Can you work these out from the model? Positions are in its coordinate system, mm. Face numbers are marked on the shaded views. Coordinates: 2 decimals unless noted, no trailing zeros. Order: outer loops, then holes, each group sorted by start corner. A loop starts at its lowest first (then second) coordinate and runs counter-clockwise, first axis right, second up. Notation, with made-up numbers: M -15,43.5 L -8,43.5 A12 ccw -8,62.5 Z; hole C 77,63 d6. An arc over 180 degrees is marked long. Answer as a JSON object with one key per item and string values.
from build123d import *

# Parameters (mm, degrees)
F0_W          = 3
F0_H          = 9
F0_H_2        = 7
F0_H_3        = 3
F0_R          = 2.1
F0_W_2        = 1
F1_DEPTH      = 2
F2_DEPTH      = 34
F3_W          = 4
F3_H          = 2
F4_DEPTH      = 34
F5_SIZE       = 1.99999
F7_W          = 1
F7_H          = 1
F8_DEPTH      = 1
F3_W_2        = 31
F9_DEPTH      = 10
F10_R         = 1.99999
F11_T1_DEPTH  = 32
F11_T3_DEPTH  = 34.50001
F11_T5_DEPTH  = 32.00001
F11_T7_DEPTH  = 19.5
F11_T9_DEPTH  = 11.5
F11_T11_DEPTH = 44
F11_T13_DEPTH = 36.5
F11_T16_ANGLE = 90
F11_T18_ANGLE = 90
F11_T23_DEPTH = 34.50001
F11_T27_DEPTH = 22
F11_T34_DEPTH = 14
F11_T38_DEPTH = 39
F11_T45_DEPTH = 22
F11_T49_DEPTH = 34.50001


# Not quite as in the source:
# - a fillet or chamfer that OpenCascade refuses, or shapes differently, is made with other operations: its cross-section is extruded or revolved along the edge and cut away or added
# - a fillet or chamfer is up to 0.001 mm smaller than in the source, because OpenCascade refuses the exact size
# - a feature of the source that left no trace in its solid (it failed there, or was rolled back) is left out
# - a feature names something its author has since deleted; it is built from what else it names


with BuildPart() as f1:
    # F0 (on Top) → F1 (new body)
    with BuildSketch(Plane.XY):
        with Locations((18, 20.5)):
            Rectangle(F0_W, F0_H)
        with Locations((-18, 20.5)):
            Rectangle(F0_W, F0_H)
        with Locations((18, -21.5)):
            Rectangle(F0_W, F0_H_2)
        with Locations((-18, -21.5)):
            Rectangle(F0_W, F0_H_2)
        with Locations((18, -16.5)):
            Rectangle(F0_W, F0_H_3)
        with Locations((-18, -16.5)):
            Rectangle(F0_W, F0_H_3)
        Polygon((19.5, -35), (19.5, -25), (16.5, -25), (-16.5, -25), (-19.5, -25), (-19.5, -35), align=None)
        with Locations((0, -30)):
            Circle(F0_R, mode=Mode.SUBTRACT)
        Polygon((19.5, -15), (19.5, 16), (16.5, 16), (16.5, 15), (16.5, -15), align=None)
        Polygon((-16.5, 15), (-16.5, 16), (-19.5, 16), (-19.5, 15), (-19.5, -15), (-16.5, -15), align=None)
        Polygon((16.5, 16), (16.5, 25), (-16.5, 25), (-16.5, 16), (-16.5, 15), (16.5, 15), align=None)
        with Locations((0, 20)):
            Circle(F0_R, mode=Mode.SUBTRACT)
        Polygon((16.5, -15), (16.5, 15), (-16.5, 15), (-16.5, -15), (-15.5, -15), (15.5, -15), align=None)
        with Locations((-16, -16.5)):
            Rectangle(F0_W_2, F0_H_3)
        with Locations((16, -16.5)):
            Rectangle(F0_W_2, F0_H_3)
        Polygon((16.5, -25), (16.5, -18), (15.5, -18), (15.5, -15), (-15.5, -15), (-15.5, -18), (-16.5, -18), (-16.5, -25), align=None)
        with Locations((0, -20)):
            Circle(F0_R, mode=Mode.SUBTRACT)
        with Locations((0, -20)):
            Circle(F0_R)
    extrude(amount=-F1_DEPTH)

    # F0 (on Top) → F2 (join)
    with BuildSketch(Plane.XY):
        Polygon((-16.5, 15), (-16.5, 16), (-19.5, 16), (-19.5, 15), (-19.5, -15), (-16.5, -15), align=None)
        with Locations((-18, -16.5)):
            Rectangle(F0_W, F0_H_3)
        with Locations((18, -16.5)):
            Rectangle(F0_W, F0_H_3)
        with Locations((16, -16.5)):
            Rectangle(F0_W_2, F0_H_3)
        with Locations((-16, -16.5)):
            Rectangle(F0_W_2, F0_H_3)
        Polygon((19.5, -15), (19.5, 16), (16.5, 16), (16.5, 15), (16.5, -15), align=None)
    extrude(amount=F2_DEPTH)

    # F3 (on face) → F4 (join)
    with BuildSketch(Plane.XZ.offset(18)):
        with Locations((-17.5, 33)):
            Rectangle(F3_W, F3_H)
        with Locations((17.5, 33)):
            Rectangle(F3_W, F3_H)
    extrude(amount=-F4_DEPTH)

    # F5 (size 2 in the source; OpenCascade refuses exactly that, so slightly less here)
    f5_edges = [f1.edges().sort_by_distance(p)[0] for p in [
        (-2.1, -30, 0),
        (-2.1, 20, 0),
    ]]
    chamfer(f5_edges, length=F5_SIZE)

    # F7 (on face) → F8 (join)
    with BuildSketch(Plane(origin=(0, 16, 0), x_dir=(-1, 0, 0), z_dir=(0, 1, 0))):
        with Locations((-16, 31.5)):
            Rectangle(F7_W, F7_H)
        Polygon((15.9987417102, 33.0025165796), (15.5, 34), (15.5050715785, 33.0000128605), align=None)
    extrude(amount=-F8_DEPTH)

    # F3 (on face) → F9 (join)
    with BuildSketch(Plane.XZ.offset(18)):
        with Locations((0, 33)):
            Rectangle(F3_W_2, F3_H)
    extrude(amount=-F9_DEPTH)

    # F10 (radius 2 in the source; OpenCascade refuses exactly that, so slightly less here)
    f10_edges = [f1.edges().sort_by_distance(p)[0] for p in [
        (0, -18, 34),
        (-15.5, 4, 34),
        (0, -8, 34),
        (15.5, 4, 34),
    ]]
    fillet(f10_edges, radius=F10_R)

    # F11: fillet of radius 1 on 15 edges, made by hand

    # F11_s2 → F11_t1 (cut)
    with BuildSketch(Plane.XY):
        with BuildLine():
            ThreePointArc((-16.5, -18), (-15.7928932188, -17.7071067812), (-15.5, -17))
            Line((-15.5, -17), (-15.5, -18))
            Line((-15.5, -18), (-16.5, -18))
        make_face()
        with BuildLine():
            ThreePointArc((15.5, -17), (15.7928932188, -17.7071067812), (16.5, -18))
            Line((16.5, -18), (15.5, -18))
            Line((15.5, -18), (15.5, -17))
        make_face()
    extrude(amount=F11_T1_DEPTH, mode=Mode.SUBTRACT)

    # F11_s4 → F11_t3 (cut)
    with BuildSketch(Plane.XZ.offset(-18.5)):
        with BuildLine():
            ThreePointArc((-18.5, 34), (-19.2071067812, 33.7071067812), (-19.5, 33))
            Line((-19.5, 33), (-19.5, 34))
            Line((-19.5, 34), (-18.5, 34))
        make_face()
        with BuildLine():
            ThreePointArc((18.5, 34), (19.2071067812, 33.7071067812), (19.5, 33))
            Line((19.5, 33), (19.5, 34))
            Line((19.5, 34), (18.5, 34))
        make_face()
    extrude(amount=F11_T3_DEPTH, mode=Mode.SUBTRACT)

    # F11_s6 → F11_t5 (cut)
    with BuildSketch(Plane.XY):
        with BuildLine():
            ThreePointArc((-19.5, -17), (-19.2071067812, -17.7071067812), (-18.5, -18))
            Line((-18.5, -18), (-19.5, -18))
            Line((-19.5, -18), (-19.5, -17))
        make_face()
        with BuildLine():
            ThreePointArc((18.5, -18), (19.2071067812, -17.7071067812), (19.5, -17))
            Line((19.5, -17), (19.5, -18))
            Line((19.5, -18), (18.5, -18))
        make_face()
    extrude(amount=F11_T5_DEPTH, mode=Mode.SUBTRACT)

    # F11_s8 → F11_t7 (cut)
    with BuildSketch(Plane.XZ.offset(18)):
        with BuildLine():
            ThreePointArc((-19.5, -1), (-19.2071067812, -0.2928932188), (-18.5, 0))
            Line((-18.5, 0), (-19.5, 0))
            Line((-19.5, 0), (-19.5, -1))
        make_face()
        with BuildLine():
            ThreePointArc((18.5, 0), (19.2071067812, -0.2928932188), (19.5, -1))
            Line((19.5, -1), (19.5, 0))
            Line((19.5, 0), (18.5, 0))
        make_face()
    extrude(amount=F11_T7_DEPTH, mode=Mode.SUBTRACT)

    # F11_s10 → F11_t9 (cut)
    with BuildSketch(Plane.XZ.offset(-27.5)):
        with BuildLine():
            ThreePointArc((-19.5, -1), (-19.2071067812, -0.2928932188), (-18.5, 0))
            Line((-18.5, 0), (-19.5, 0))
            Line((-19.5, 0), (-19.5, -1))
        make_face()
        with BuildLine():
            ThreePointArc((18.5, 0), (19.2071067812, -0.2928932188), (19.5, -1))
            Line((19.5, -1), (19.5, 0))
            Line((19.5, 0), (18.5, 0))
        make_face()
    extrude(amount=F11_T9_DEPTH, mode=Mode.SUBTRACT)

    # F11_s12 → F11_t11 (cut)
    with BuildSketch(Plane.YZ.offset(-22)):
        with BuildLine():
            ThreePointArc((-34, 0), (-34.7071067812, -0.2928932188), (-35, -1))
            Line((-35, -1), (-35, 0))
            Line((-35, 0), (-34, 0))
        make_face()
        with BuildLine():
            ThreePointArc((24, 0), (24.7071067812, -0.2928932188), (25, -1))
            Line((25, -1), (25, 0))
            Line((25, 0), (24, 0))
        make_face()
    extrude(amount=F11_T11_DEPTH, mode=Mode.SUBTRACT)

    # F11_s14 → F11_t13 (cut)
    with BuildSketch(Plane.XY):
        with BuildLine():
            ThreePointArc((19.5, 15), (19.2071067812, 15.7071067812), (18.5, 16))
            Line((18.5, 16), (19.5, 16))
            Line((19.5, 16), (19.5, 15))
        make_face()
    extrude(amount=F11_T13_DEPTH, mode=Mode.SUBTRACT)

    # F11_s15 → F11_t16 (revolve, cut)
    with BuildSketch(Plane.XZ.offset(16.00001)):
        with BuildLine():
            ThreePointArc((-19.5, 33), (-19.2071067812, 33.7071067812), (-18.5, 34))
            Line((-18.5, 34), (-19.5, 34))
            Line((-19.5, 34), (-19.5, 33))
        make_face()
    revolve(axis=Axis((-19.5, -16.00001, 32.00001), (1, 0, 0)), revolution_arc=F11_T16_ANGLE, mode=Mode.SUBTRACT)

    # F11_s17 → F11_t18 (revolve, cut)
    with BuildSketch(Plane.XZ.offset(16.00001)):
        with BuildLine():
            ThreePointArc((18.5, 34), (19.2071067812, 33.7071067812), (19.5, 33))
            Line((19.5, 33), (19.5, 34))
            Line((19.5, 34), (18.5, 34))
        make_face()
    revolve(axis=Axis((19.5, -16.00001, 32.00001), (1, 0, 0)), revolution_arc=F11_T18_ANGLE, mode=Mode.SUBTRACT)


with BuildPart() as f11_tool21:
    # F11_s22 → F11_t23 (new body)
    with BuildSketch(Plane.XY.offset(-2.5)):
        with BuildLine():
            ThreePointArc((-19.5, -17), (-19.2071067812, -17.7071067812), (-18.5, -18))
            Line((-18.5, -18), (-19.5, -18))
            Line((-19.5, -18), (-19.5, -17))
        make_face()
    extrude(amount=F11_T23_DEPTH)

    split(bisect_by=Plane.XY, keep=Keep.BOTTOM)


with BuildPart() as f11_tool25:
    # F11_s26 → F11_t27 (new body)
    with BuildSketch(Plane.XZ.offset(15.5)):
        with BuildLine():
            ThreePointArc((-19.5, -1), (-19.2071067812, -0.2928932188), (-18.5, 0))
            Line((-18.5, 0), (-19.5, 0))
            Line((-19.5, 0), (-19.5, -1))
        make_face()
    extrude(amount=F11_T27_DEPTH)

    split(bisect_by=Plane.XZ.offset(18), keep=Keep.BOTTOM)


with BuildPart() as f11_tool21_1:
    add(f11_tool21.part)

    # F11_t29: intersect F11_tool25
    add(f11_tool25.part, mode=Mode.INTERSECT)


with BuildPart() as f1_1:
    add(f1.part)

    # F11_t19: cut F11_tool21
    add(f11_tool21_1.part, mode=Mode.SUBTRACT)


with BuildPart() as f11_tool32:
    # F11_s33 → F11_t34 (new body)
    with BuildSketch(Plane.XZ.offset(-13.5)):
        with BuildLine():
            ThreePointArc((18.5, 0), (19.2071067812, -0.2928932188), (19.5, -1))
            Line((19.5, -1), (19.5, 0))
            Line((19.5, 0), (18.5, 0))
        make_face()
    extrude(amount=-F11_T34_DEPTH)

    split(bisect_by=Plane.XZ.offset(-16), keep=Keep.TOP)


with BuildPart() as f11_tool36:
    # F11_s37 → F11_t38 (new body)
    with BuildSketch(Plane.XY.offset(-2.5)):
        with BuildLine():
            ThreePointArc((19.5, 15), (19.2071067812, 15.7071067812), (18.5, 16))
            Line((18.5, 16), (19.5, 16))
            Line((19.5, 16), (19.5, 15))
        make_face()
    extrude(amount=F11_T38_DEPTH)

    split(bisect_by=Plane.XY, keep=Keep.BOTTOM)


with BuildPart() as f11_tool32_1:
    add(f11_tool32.part)

    # F11_t40: intersect F11_tool36
    add(f11_tool36.part, mode=Mode.INTERSECT)


with BuildPart() as f1_2:
    add(f1_1.part)

    # F11_t30: cut F11_tool32
    add(f11_tool32_1.part, mode=Mode.SUBTRACT)


with BuildPart() as f11_tool43:
    # F11_s44 → F11_t45 (new body)
    with BuildSketch(Plane.XZ.offset(37.5)):
        with BuildLine():
            ThreePointArc((18.5, 0), (19.2071067812, -0.2928932188), (19.5, -1))
            Line((19.5, -1), (19.5, 0))
            Line((19.5, 0), (18.5, 0))
        make_face()
    extrude(amount=-F11_T45_DEPTH)

    split(bisect_by=Plane.XZ.offset(18), keep=Keep.BOTTOM)


with BuildPart() as f11_tool47:
    # F11_s48 → F11_t49 (new body)
    with BuildSketch(Plane.XY.offset(32.00001)):
        with BuildLine():
            ThreePointArc((18.5, -18), (19.2071067812, -17.7071067812), (19.5, -17))
            Line((19.5, -17), (19.5, -18))
            Line((19.5, -18), (18.5, -18))
        make_face()
    extrude(amount=-F11_T49_DEPTH)

    split(bisect_by=Plane.XY, keep=Keep.BOTTOM)


with BuildPart() as f11_tool43_1:
    add(f11_tool43.part)

    # F11_t51: intersect F11_tool47
    add(f11_tool47.part, mode=Mode.INTERSECT)


with BuildPart() as f1_3:
    add(f1_2.part)

    # F11_t41: cut F11_tool43
    add(f11_tool43_1.part, mode=Mode.SUBTRACT)


solid = f1_3.part
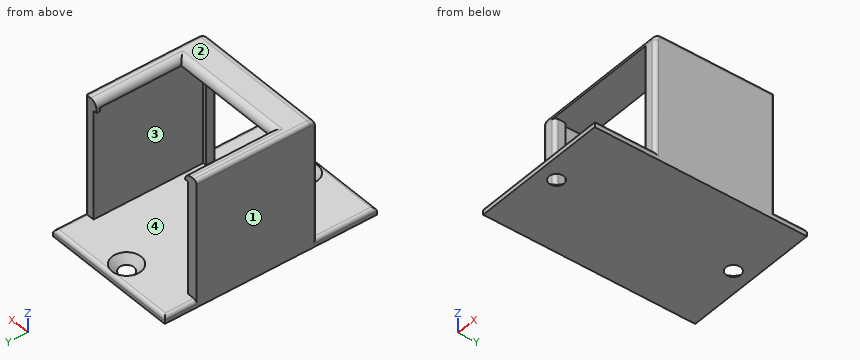
Item 1: I'm going to push flat-ended pins straight in: pin 1 (0.8 mm diameter, centred on x = 16, z = 18.5, fed in from +Y); pin 2 (4.5 mm diameter, centred on x = -18.5, z = 11, fed in from +Y); pin 3 (4 mm diameter, centred on x = 0, y = 20, fed in from +Z); pin 4 (16 mm diameter, centred on x = -9, z = 13, fed in from -Y). Where does each tip first touch, or does it pass through?
Answers follow:
{"pin 1": "stops at y = -15", "pin 2": "stops at y = 16", "pin 3": "passes through", "pin 4": "stops at y = -18"}
Item 2: If we mould it in two halves opening along X, with no side actions, what happens to the marked faces 1, 2, 3 and 4? For each: pulls with the +X half, pulls with the -X half, needs draft (parallel to the pull), parting line crosses it, or undercut.
Answers follow:
{"face 1": "pulls with the -X half", "face 2": "needs draft", "face 3": "undercut", "face 4": "undercut"}
Item 3: Please list where these lines run through material, in increasing order: line 1 (X direction, y = 4, z = 25); line 2 (Y direction, x = 0, z = -1.95); line 3 (Z direction, x = -3.5, y = -15).
Answers follow:
{"line 1": "x = -19.5 to -16.5, 16.5 to 19.5", "line 2": "y = -35 to -32.15, -27.85 to 17.85, 22.15 to 25", "line 3": "z = -2 to 0, 32 to 34"}
Item 4: I want a section at B-B, the plane z = 14. Write out the boundary of the cut face in (x, y), plus the area to 3 significant figures.
Answers follow:
{"outline": "M -19.5,-17 A1 ccw -18.5,-18 L -16.5,-18 A1 ccw -15.5,-17 L -15.5,-15 L -16.5,-15 L -16.5,16 L -19.5,16 Z; M 15.5,-17 A1 ccw 16.5,-18 L 18.5,-18 A1 ccw 19.5,-17 L 19.5,15 A1 ccw 18.5,16 L 16.5,16 L 16.5,-15 L 15.5,-15 Z", "area": "209 mm^2"}
Item 5: I want a section at D-D, the plane x = 0. Give the number of separate pieces and of enclosed holes in the cut face, plus the area to 3 significant figures.
Answers follow:
{"separate pieces": "4", "enclosed holes": "0", "area": "113 mm^2"}
